For this review, take the finished solid that the model builds, in its own axes (mm). Face numbers are marked on the shaded views. A direction names the side the tool comes from. Round coordinates to 2 decimals unless told otherwise and drop trailing zeros. Write each loop counter-clockwise with the first axis right and the second up, starting at its lowest first coordinate (ties: lowest second). Pieces come first, ordered by that corner, then holes. Notation, with made-up numbers: M -24,19 L -13,19 A22 cw -13,41 Z; hole C 53,75.5 d2. An arc over 180 degrees is marked long. Answer in a Markdown table with one row per item.
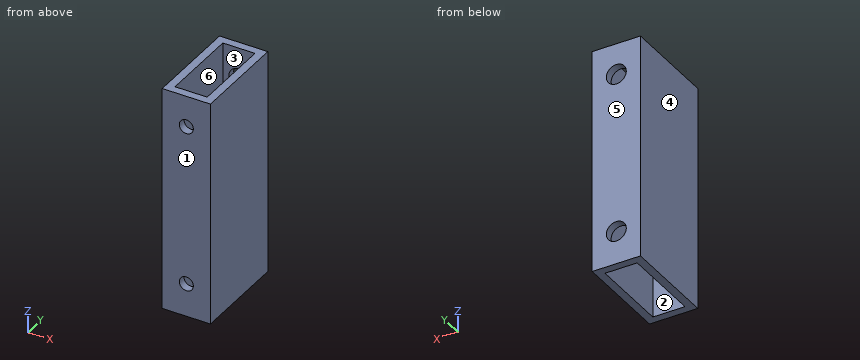
```python
from build123d import *

# Parameters (mm, degrees)
SKETCH1_W           = 19.05
SKETCH1_H           = 38.1
SKETCH1_W_2         = 12.7
SKETCH1_H_2         = 31.75
BOSS_EXTRUDE1_DEPTH = 88.9
SKETCH2_R           = 2.778125
CUT_EXTRUDE1_DEPTH  = 98.188196943
CUT_EXTRUDE2_REACH  = 99.188
SKETCH3_R           = 3.937


with BuildPart() as part:
    # Sketch1 → Boss-Extrude1 (new body)
    with BuildSketch(Plane.XY):
        Rectangle(SKETCH1_W, SKETCH1_H)
        Rectangle(SKETCH1_W_2, SKETCH1_H_2, mode=Mode.SUBTRACT)
    extrude(amount=BOSS_EXTRUDE1_DEPTH)

    # Sketch2 → Cut-Extrude1 (cut, through all)
    with BuildSketch(Plane(origin=(0, 19.05, 0), x_dir=(1, 0, 0), z_dir=(0, 1, 0))):
        with Locations(Location((0, -76.596875, 0), (0, 0, 270))):
            Circle(SKETCH2_R)
        with Locations(Location((0, -13.096875, 0), (0, 0, 270))):
            Circle(SKETCH2_R)
    extrude(amount=-CUT_EXTRUDE1_DEPTH, mode=Mode.SUBTRACT)

    # Sketch3 → Cut-Extrude2 (cut, up to next)
    with BuildSketch(Plane(origin=(0, 19.05, 0), x_dir=(1, 0, 0), z_dir=(0, 1, 0)), mode=Mode.PRIVATE) as cut_extrude2_sk1:
        with Locations(Location((0, -76.596875, 0), (0, 0, 270))):
            Circle(SKETCH3_R)
    cut_extrude2_tool1 = extrude(cut_extrude2_sk1.sketch, amount=-CUT_EXTRUDE2_REACH, mode=Mode.PRIVATE) & part.part
    # Sketch3 → Cut-Extrude2 (cut, up to next)
    with BuildSketch(Plane(origin=(0, 19.05, 0), x_dir=(1, 0, 0), z_dir=(0, 1, 0)), mode=Mode.PRIVATE) as cut_extrude2_sk2:
        with Locations(Location((0, -13.096875, 0), (0, 0, 270))):
            Circle(SKETCH3_R)
    cut_extrude2_tool2 = extrude(cut_extrude2_sk2.sketch, amount=-CUT_EXTRUDE2_REACH, mode=Mode.PRIVATE) & part.part
    add(cut_extrude2_tool1.solids().sort_by_distance((0, 19.05, 76.596875))[0], mode=Mode.SUBTRACT)
    add(cut_extrude2_tool2.solids().sort_by_distance((0, 19.05, 13.096875))[0], mode=Mode.SUBTRACT)


solid = part.part
```
Q1. Take a section at B-B (y = -0.5). State the section outline as (x, z) points (3 decimals).
Found:
| item | result |
|---|---|
| outline | M -9.525,0 L -6.35,0 L -6.35,88.9 L -9.525,88.9 Z; M 6.35,0 L 9.525,0 L 9.525,88.9 L 6.35,88.9 Z |
Q2. Insertion check: P1, Ø5, axis at x = 0, z = 76.6, coming from the +Y side. The pin has a flat end and moves straight along its axis. Give the tip position at first contact, or say it passes through.
Found:
| item | result |
|---|---|
| P1 | through |
Q3. Take a section at A-A (x = 0). State the section outline as (y, z) points (3 decimals).
Found:
| item | result |
|---|---|
| outline | M -19.05,0 L -15.875,0 L -15.875,10.319 L -19.05,10.319 Z; M -19.05,15.875 L -15.875,15.875 L -15.875,73.819 L -19.05,73.819 Z; M -19.05,79.375 L -15.875,79.375 L -15.875,88.9 L -19.05,88.9 Z; M 15.875,0 L 19.05,0 L 19.05,9.16 L 15.875,9.16 Z; M 15.875,17.034 L 19.05,17.034 L 19.05,72.66 L 15.875,72.66 Z; M 15.875,80.534 L 19.05,80.534 L 19.05,88.9 L 15.875,88.9 Z |
Q4. Machinability: for the marked faces 1 and 2, which of the approach directions +Z, -Z, +X, -X, +Y, -Y give a long, thin tool a straight path to every point of the face, cutting with its end or side? Answer none if there is none.
Found:
| item | result |
|---|---|
| face 1 | +Z, -Z, +X, -X, -Y |
| face 2 | +Z, -Z |
Q5. For probe 1 along X at (y, z) = (6.5, 6.5) (3 decimals); probe 2 along Y at (x, z) = (6.25, 50) (3 decimals); probe 3 along Y at (x, z) = (-0.25, 16) (3 decimals), list the stretches that pass through material, from the lowest coordinate up.
Found:
| item | result |
|---|---|
| probe 1 | -9.525 to -6.35, 6.35 to 9.525 |
| probe 2 | -19.05 to -15.875, 15.875 to 19.05 |
| probe 3 | -19.05 to -15.875 |
Q6. Take a section at C-C (z = 28). State the section outline as (x, y) points (3 decimals), then the cut area to 3 significant figures.
Found:
| item | result |
|---|---|
| outline | M -9.525,-19.05 L 9.525,-19.05 L 9.525,19.05 L -9.525,19.05 Z; hole M -6.35,-15.875 L 6.35,-15.875 L 6.35,15.875 L -6.35,15.875 Z |
| area | 323 mm² |
Q7. Mouldability with a two-part tool opening along Y and no side actions: class the marked faces 3, 4, 5 and 6 as +Y half, -Y half, draft (parallel to the pull), parting line (faces both ways), or undercut.
Found:
| item | result |
|---|---|
| face 3 | undercut |
| face 4 | draft |
| face 5 | +Y half |
| face 6 | undercut |
